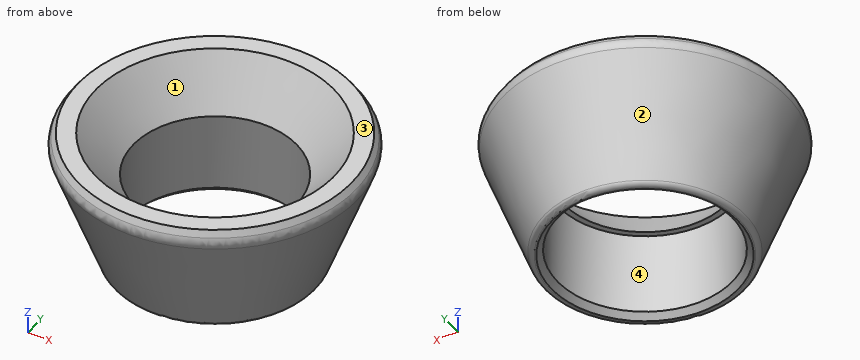
```python
from build123d import *

# Parameters (mm, degrees)
F2_SIZE = 2
F3_R    = 2
F4_SIZE = 1
F5_R    = 1


with BuildPart() as f1:
    # F0 (on Front) → F1 (revolve)
    with BuildSketch(Plane.XZ):
        Polygon((15, 15), (15, 0), (17, 0), (25.4278760969, 22.6604444312), (20.4278760969, 22.6604444312), (14, 15), align=None)
    revolve(axis=Axis((0, 0, 7.5), (0, 0, 1)))

    # F2
    f2_edges = [f1.edges().sort_by_distance(p)[0] for p in [
        (-25.427876, 0, 22.660444),
    ]]
    chamfer(f2_edges, length=F2_SIZE)

    # F3
    f3_edges = [f1.edges().sort_by_distance(p)[0] for p in [
        (-24.730693, 0, 20.785895),
    ]]
    fillet(f3_edges, radius=F3_R)

    # F4
    f4_edges = [f1.edges().sort_by_distance(p)[0] for p in [
        (-15, 0, 0),
    ]]
    chamfer(f4_edges, length=F4_SIZE)

    # F5
    f5_edges = [f1.edges().sort_by_distance(p)[0] for p in [
        (-17, 0, 0),
    ]]
    fillet(f5_edges, radius=F5_R)


solid = f1.part
```
Source: CAD feature listing. Evaluate the final solid. Frame: model axes, mm. Face numbers are marked on the shaded views. Round coordinates to 2 decimals unless told otherwise and drop trailing zeros. Write each loop counter-clockwise with the first axis right and the second up, starting at its lowest first coordinate (ties: lowest second). Pieces come first, ordered by that corner, then holes. Notation, with made-up numbers: M 61.5,42 L 109.5,42 A30 ccw 109.5,67 Z; hole C -37.5,82 d7. An arc over 180 degrees is marked long. Answer as a JSON object with one key per item and string values. Group by question number.
(1) First-contact query: pin 1 (6 mm diameter, centred on y = 18.5, z = 4.5, fed in from -X); pin 2 (1.5 mm diameter, centred on x = 3.5, z = 7, fed in from -Y); pin 3 (6 mm diameter, centred on x = -4, z = 17.5, fed in from +Y). Flat tips, straight axial feed; report the tip coordinate or a pass-through.
(2) Section query A-A on z = 13. Output: boundary loops of the cut face in (x, y), then the cut area to 3 significant figures.
(3) Mould query, pull axis X, two halves, no side actions, for the marked faces 1, 2, 3 and 4. Classes: +X half, -X half, draft (parallel to the pull), parting line (faces both ways), or undercut.
(4) Section query B-B on z = 3.5. Output: boundary loops of the cut face in (x, y).
(5) Ray query, line 1 (Y direction, x = 5.5, z = 7.75); line 2 (Y direction, x = 0, z = 8.75); line 3 (X direction, y = -13, z = 12). Return the intervals inside material, ascending. Write a range as [from, to].
Computed values:
{
 "1": {"pin 1": "x = -10.84", "pin 2": "y = -19.6", "pin 3": "y = 24.32"},
 "2": {"outline": "C 0,0 d43.67; hole C 0,0 d30", "area": "791 mm^2"},
 "3": {"face 1": "undercut", "face 2": "parting line", "face 3": "draft", "face 4": "undercut"},
 "4": {"outline": "C 0,0 d36.6; hole C 0,0 d30"},
 "5": {"line 1": "[-19.11, -13.96], [13.96, 19.11]", "line 2": "[-20.25, -15], [15, 20.25]", "line 3": "[-17.08, -7.48], [7.48, 17.08]"}
}
